```python
from build123d import *

# Parameters (mm, degrees)
SKETCH1_W           = 22.5
SKETCH1_H           = 32
BOSS_EXTRUDE1_DEPTH = 2
BOSS_EXTRUDE3_START = -2
BOSS_EXTRUDE3_DEPTH = 7


with BuildPart() as part:
    # Sketch1 → Boss-Extrude1 (new body)
    with BuildSketch(Plane(origin=(0, 0, 0), x_dir=(1, 0, 0), z_dir=(0, 1, 0))):
        Rectangle(SKETCH1_W, SKETCH1_H)
    extrude(amount=BOSS_EXTRUDE1_DEPTH)

    # Sketch3 → Boss-Extrude3 (add)
    with BuildSketch(Plane(origin=(0, 2, 0), x_dir=(1, 0, 0), z_dir=(0, 1, 0)).offset(BOSS_EXTRUDE3_START)):
        Polygon((-11.25, -16), (-11.25, 16), (11.25, 16), (11.25, -16), (13.25, -16), (13.25, 18), (-13.25, 18), (-13.25, -16), align=None)
    extrude(amount=BOSS_EXTRUDE3_DEPTH)


solid = part.part
```
Check sheet for the modelled part. Datum: model origin and axes. Units: mm. A direction names the side the tool comes from. Give positions to 0.01 mm unless a question says otherwise; leave off trailing zeros. Loops run counter-clockwise (first coordinate to the right, second up) from the corner with the lowest first, then second, coordinate; pieces in that order, holes last. Notation, with made-up numbers: M 56.25,77 L 65.25,77 A17 cw 65.25,98 Z; hole C 30.25,8 d8. An arc over 180 degrees is marked long. Answer in a Markdown table with one row per item.
1) Cross-section at C-C (x = -9.75). Enter the section's corners in (y, z).
Solutions:
| item | result |
|---|---|
| outline | M 0,-18 L 7,-18 L 7,-16 L 2,-16 L 2,16 L 0,16 Z |
2) Cross-section at A-A (y = 3). Enter the section's corners in (x, z), plus the area to 3 significant figures.
Solutions:
| item | result |
|---|---|
| outline | M -13.25,-18 L 13.25,-18 L 13.25,16 L 11.25,16 L 11.25,-16 L -11.25,-16 L -11.25,16 L -13.25,16 Z |
| area | 181 mm^2 |
3) Mould release check, pull along X, two halves, no side actions. Record for faces 3 (the face through (-13.25, 3, -1)), 4 (the face through (0, 2, 0)), 5 (the face through (13.25, 3, -1)), 6 (the face through (0, 1, 16)): released by +X, released by -X, zero draft, split by the parting line, or undercut.
Solutions:
| item | result |
|---|---|
| face 3 | released by -X |
| face 4 | undercut |
| face 5 | released by +X |
| face 6 | zero draft |
4) Thickness scan on line 1 (X direction, y = 6, z = -7); line 2 (Y direction, x = 10.5, z = 6); line 3 (Z direction, x = -9, y = 3). Record the ranges inside material, lowest first.
Solutions:
| item | result |
|---|---|
| line 1 | x = -13.25 to -11.25, 11.25 to 13.25 |
| line 2 | y = 0 to 2 |
| line 3 | z = -18 to -16 |
5) Cross-section at B-B (z = -14.5). Enter the section's corners in (x, y), plus the area to 3 significant figures.
Solutions:
| item | result |
|---|---|
| outline | M -13.25,0 L 13.25,0 L 13.25,7 L 11.25,7 L 11.25,2 L -11.25,2 L -11.25,7 L -13.25,7 Z |
| area | 73.0 mm^2 |
6) Tool access check on faces 1 (the face through (11.25, 4, 0)), 2 (the face through (0, 3, -18)). Record the directions out of +Z, -Z, +X, -X, +Y, -Y that give a thin tool (end or side, any length) a straight path to the whole face; none if there is none.
Solutions:
| item | result |
|---|---|
| face 1 | +Z, +Y |
| face 2 | -Z, +X, -X, +Y, -Y |
7) Depth check by flat-ended pin: pin 1 (4 mm diameter, centred on x = -4.5, y = 5.5, fed in from +Z); pin 2 (3 mm diameter, centred on x = -0.5, z = 3, fed in from +Y). Enter the tip coordinate at first touch or a pass-through.
Solutions:
| item | result |
|---|---|
| pin 1 | stops at z = -16 |
| pin 2 | stops at y = 2 |
